Build history of the part. All positions in model axes, mm. Face numbers are marked on the shaded views. A direction names the side the tool comes from. Round coordinates to 2 decimals unless told otherwise and drop trailing zeros. Order: outer loops, then holes, each group sorted by start corner. A loop starts at its lowest first (then second) coordinate and runs counter-clockwise, first axis right, second up. Notation, with made-up numbers: (9, 32.5) -> (45, 32.5) arc R15 ccw to (45, 36.5) -> close; hole circle Ø4 at (59.5, -40). An arc over 180 degrees is marked (long way). Write item = value, one per line.
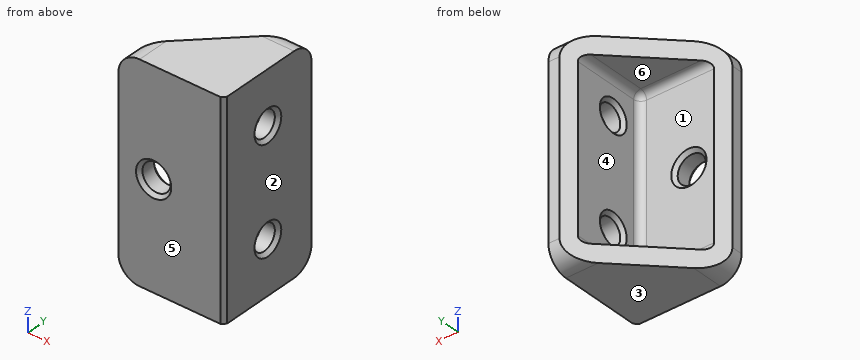
from build123d import *

# Parameters (mm, degrees)
BOSS_EXTRUDE1_DEPTH = 30
CUT_EXTRUDE1_START  = -2.5
CUT_EXTRUDE1_DEPTH  = 25
SKETCH4_R           = 1.8
CUT_EXTRUDE2_DEPTH  = 25
FILLET1_R           = 1
FILLET2_R           = 3
SKETCH5_R           = 2
CUT_EXTRUDE3_DEPTH  = 25
CUT_EXTRUDE4_DEPTH  = 37.742346142
CHAMFER1_SIZE       = 0.5


with BuildPart() as part:
    # Sketch1 → Boss-Extrude1 (new body)
    with BuildSketch(Plane.XY):
        Polygon((0, 0), (0, 15), (-3, 15), (-15, 3), (-15, 0), align=None)
    extrude(amount=BOSS_EXTRUDE1_DEPTH)

    # Sketch3 → Cut-Extrude1 (cut)
    with BuildSketch(Plane.XY.offset(30).offset(CUT_EXTRUDE1_START)):
        Polygon((-15, 3), (-3, 3), (-3, 15), align=None)
    extrude(amount=-CUT_EXTRUDE1_DEPTH, mode=Mode.SUBTRACT)

    # Sketch4 → Cut-Extrude2 (cut)
    with BuildSketch(Plane.ZY.offset(3)):
        with Locations((7.5, 7.5)):
            Circle(SKETCH4_R)
        with Locations((22.5, 7.5)):
            Circle(SKETCH4_R)
    extrude(amount=-CUT_EXTRUDE2_DEPTH, mode=Mode.SUBTRACT)

    # Fillet1
    fillet1_edges = [part.edges().sort_by_distance(p)[0] for p in [
        (-3, 9, 2.5),
        (-9, 3, 2.5),
        (-3, 3, 15),
        (-9, 3, 27.5),
        (-3, 9, 27.5),
    ]]
    fillet(fillet1_edges, radius=FILLET1_R)

    # Fillet2
    fillet2_edges = [part.edges().sort_by_distance(p)[0] for p in [
        (-1.5, 15, 30),
        (-15, 1.5, 30),
        (-15, 1.5, 0),
        (-1.5, 15, 0),
    ]]
    fillet(fillet2_edges, radius=FILLET2_R)

    # Sketch5 → Cut-Extrude3 (cut)
    with BuildSketch(Plane(origin=(0, 3, 0), x_dir=(1, 0, 0), z_dir=(0, 1, 0))):
        with Locations(Location((-10, -15, 0), (0, 0, 270))):
            Circle(SKETCH5_R)
    extrude(amount=-CUT_EXTRUDE3_DEPTH, mode=Mode.SUBTRACT)

    # Sketch6 → Cut-Extrude4 (cut, through all)
    with BuildSketch(Plane(origin=(0, 0, 0), x_dir=(-1, 0, 0), z_dir=(0, 0, -1))):
        Polygon((-1.604036942, 18.18982338), (17.835092671, -1.249306233), (19.956413015, 0.87201411), (-1.074092092, 21.902519217), align=None)
    extrude(amount=-CUT_EXTRUDE4_DEPTH, mode=Mode.SUBTRACT)

    # Chamfer1
    chamfer1_edges = [part.edges().sort_by_distance(p)[0] for p in [
        (0, 7.5, 5.7),
        (-3, 7.5, 5.7),
        (0, 7.5, 20.7),
        (-3, 7.5, 20.7),
        (-10, 0, 13),
        (-10, 3, 13),
        (0, 0, 15),
    ]]
    chamfer(chamfer1_edges, length=CHAMFER1_SIZE)


solid = part.part
Q1. Cut at A-A, the plane z = 22.5. List the corners of the cut face in (x, y).
Check values:
outline = (-15, 0) -> (-0.5, 0) -> (0, 0.5) -> (0, 5.2) -> (-0.5, 5.7) -> (-2.5, 5.7) -> (-3, 5.2) -> (-3, 4) arc R1 cw to (-4, 3) -> (-13.59, 3) -> (-15, 1.59) -> close; (-3, 9.8) -> (-2.5, 9.3) -> (-0.5, 9.3) -> (0, 9.8) -> (0, 15) -> (-1.59, 15) -> (-3, 13.59) -> close
Q2. Which spindle directions (+Z, -Z, +X, -X, +Y, -Y) get a long thin tool onto all of the face, cutting with end or side? Do the marked faces 1 and 2. Say none if no direction does.
Check values:
face_1 = -X, +Y
face_2 = +Z, -Z, +X, +Y, -Y
Q3. Cut at D-D, the plane z = 25.5. List the corners of the cut face in (x, y).
Check values:
outline = (-15, 0) -> (-0.5, 0) -> (0, 0.5) -> (0, 15) -> (-1.59, 15) -> (-3, 13.59) -> (-3, 4) arc R1 cw to (-4, 3) -> (-13.59, 3) -> (-15, 1.59) -> close
Q4. Mould opens along Z. For the marked faces 3, 4, 5 and 6 say: released by +Z, released by -Z, zero draft, split by the parting line, or undercut.
Check values:
face_3 = released by -Z
face_4 = undercut
face_5 = zero draft
face_6 = undercut
Q5. Flat gauge pins, fed straight in: pin 1 (4 mm diameter, centred on y = 7.5, z = 7.5, fed in from -X); pin 2 (3 mm diameter, centred on x = -7.5, z = 18, fed in from +Y); pin 3 (3 mm diameter, centred on y = 8, z = 11.5, fed in from -X); pin 4 (8 mm diameter, centred on x = -13, y = 13.5, fed in from -Z). Where does each tip first touch, or does it go through?
Check values:
pin_1 = -2.7
pin_2 = 3
pin_3 = -3
pin_4 = through
Q6. Probe probe 1 along Y at (x, z) = (-1.4, 7.5); probe 2 along X at (y, z) = (1.25, 15); probe 3 along X at (y, z) = (11.25, 7.5). List the from-to ranges inside material, lowest first.
Check values:
probe_1 = 0 to 5.7, 9.3 to 15
probe_2 = -15 to -12, -8 to 0
probe_3 = -3 to 0
Q7. Cut at C-C, the plane y = 7.5. List the corners of the cut face in (x, z), and give its area (3 significant figures).
Check values:
outline = (-9.09, 0) -> (0, 0) -> (0, 5.2) -> (-0.5, 5.7) -> (-2.5, 5.7) -> (-3, 5.2) -> (-3, 3.5) arc R1 cw to (-4, 2.5) -> (-9.09, 2.5) -> close; (-9.09, 27.5) -> (-4, 27.5) arc R1 cw to (-3, 26.5) -> (-3, 24.8) -> (-2.5, 24.3) -> (-0.5, 24.3) -> (0, 24.8) -> (0, 30) -> (-9.09, 30) -> close; (-3, 9.8) -> (-2.5, 9.3) -> (-0.5, 9.3) -> (0, 9.8) -> (0, 20.2) -> (-0.5, 20.7) -> (-2.5, 20.7) -> (-3, 20.2) -> close
area = 98.3 mm²
Q8. Cut at B-B, the plane x = -1.25. List the corners of the cut face in (y, z), and give its area (3 significant figures).
Check values:
outline = (0, 0) -> (12, 0) arc R3 ccw to (15, 3) -> (15, 27) arc R3 ccw to (12, 30) -> (0, 30) -> close; hole circle Ø3.6 at (7.5, 7.5); hole circle Ø3.6 at (7.5, 22.5)
area = 426 mm²
